Design review of the part built by this model. Coordinates are the model's own, in mm. Face numbers are marked on the shaded views. A direction names the side the tool comes from. Give positions to 0.01 mm unless a question says otherwise; leave off trailing zeros. Loops run counter-clockwise (first coordinate to the right, second up) from the corner with the lowest first, then second, coordinate; pieces in that order, holes last. Notation, with made-up numbers: (23, -23.5) -> (38, -23.5) arc R31 cw to (38, 4.5) -> close; hole circle Ø2 at (-25, 78.5). An arc over 180 degrees is marked (long way). Answer in a Markdown table with one row per item. Add a question column.
(1) Consider section C-C on x = -11.5. Write out the cut boundary in (y, z), then the cut area to 3 significant figures.
(2) For the marked faces 4, 5 and 6, list the 3-axis set-ups (+Z, -Z, +X, -X, +Y, -Y) from which the entire face can be reached by the end or side of a thin tool; tool diameter is ignored.
(3) Consider section A-A on z = 90. Write out the cut boundary in (x, y).
(4) Draft analysis for pull direction Y (two halves, no side actions). For the marked faces 1, 2 and 3, state which applies: +Y half, -Y half, draft (parallel to the pull), parting line (faces both ways), or undercut.
(5) Consider section D-D on z = 106. Write out the cut boundary in (x, y), then the cut area to 3 significant figures.
(6) For line 1 (Y direction, x = 34.5, z = 90.5); line 2 (Z direction, x = 6.5, y = -20); line 3 (X direction, y = 33, z = 91), list the stretches that pass through material, from the lowest coordinate up.
(7) Consider section B-B on y = 26.5. Write out the cut boundary in (x, z), then the cut area to 3 significant figures.
(8) For pin 1 (3 mm diameter, centred on x = -22.5, z = 48.5, fed in from -Y); pin 2 (11 mm diameter, centred on y = 30.5, z = 74.5, fed in from -X); pin 3 (3 mm diameter, centred on y = -30.5, z = 70.5, fed in from +X), all flat-tipped, find the tip position at first contact; note any pin that passes through.
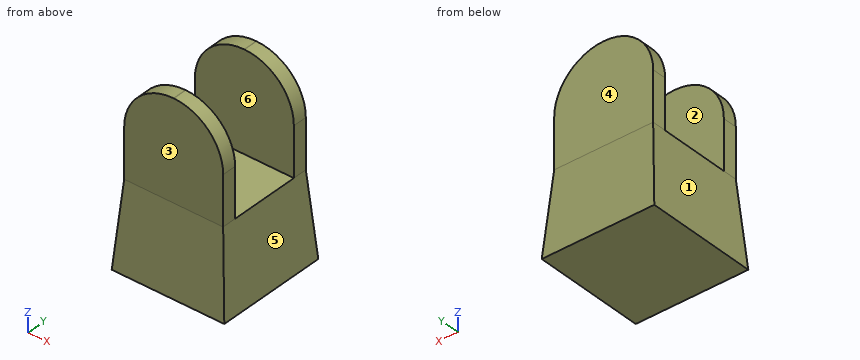
from build123d import *

# Parameters (mm, degrees)
SZKIC1_W                    = 80
SZKIC1_H                    = 80
DODANIE_WYCI_GNI_CIE1_DEPTH = 60
DODANIE_WYCI_GNI_CIE1_TAPER = 4.6
SZKIC6_W                    = 70.345029246
SZKIC6_H                    = 70.345029246
DODANIE_WYCI_GNI_CIE2_DEPTH = 70
ZAOKR_GLENIE3_R             = 35
ZAOKR_GLENIE4_R             = 35
SZKIC7_W                    = 70.345029246
SZKIC7_H                    = 50
WYTNIJ_WYCI_GNI_CIE3_DEPTH  = 70


with BuildPart() as part:
    # Szkic1 → Dodanie-wyciągnięcie1 (new body)
    with BuildSketch(Plane.XY):
        Rectangle(SZKIC1_W, SZKIC1_H)
    extrude(amount=DODANIE_WYCI_GNI_CIE1_DEPTH, taper=DODANIE_WYCI_GNI_CIE1_TAPER)

    # Szkic6 → Dodanie-wyciągnięcie2 (add)
    with BuildSketch(Plane.XY.offset(60)):
        Rectangle(SZKIC6_W, SZKIC6_H)
    extrude(amount=DODANIE_WYCI_GNI_CIE2_DEPTH)

    # Zaokrąglenie3
    zaokr_glenie3_edges = [part.edges().sort_by_distance(p)[0] for p in [
        (-35.172514623, 0, 130),
    ]]
    fillet(zaokr_glenie3_edges, radius=ZAOKR_GLENIE3_R)

    # Zaokrąglenie4
    zaokr_glenie4_edges = [part.edges().sort_by_distance(p)[0] for p in [
        (35.172514623, 0, 130),
    ]]
    fillet(zaokr_glenie4_edges, radius=ZAOKR_GLENIE4_R)

    # Szkic7 → Wytnij-wyciągnięcie3 (cut)
    with BuildSketch(Plane.XY.offset(130)):
        Rectangle(SZKIC7_W, SZKIC7_H)
    extrude(amount=-WYTNIJ_WYCI_GNI_CIE3_DEPTH, mode=Mode.SUBTRACT)


solid = part.part
Values follow:
| question | item | result |
|---|---|---|
| 1 | outline | (-40, 0) -> (40, 0) -> (35.17, 60) -> (35.17, 128.12) -> (25, 128.12) -> (25, 60) -> (-25, 60) -> (-25, 128.12) -> (-35.17, 128.12) -> (-35.17, 60) -> close |
| 1 | area | 5,900 mm2 |
| 2 | face 4 | +Z, +X, -X, +Y |
| 2 | face 5 | +Z, +X, +Y, -Y |
| 2 | face 6 | +Z, +X, -X |
| 3 | outline | (-35.17, -35.17) -> (35.17, -35.17) -> (35.17, -25) -> (-35.17, -25) -> close; (-35.17, 25) -> (35.17, 25) -> (35.17, 35.17) -> (-35.17, 35.17) -> close |
| 4 | face 1 | draft |
| 4 | face 2 | undercut |
| 4 | face 3 | -Y half |
| 5 | outline | (-33.4, -35.17) -> (33.4, -35.17) -> (33.4, -25) -> (-33.4, -25) -> close; (-33.4, 25) -> (33.4, 25) -> (33.4, 35.17) -> (-33.4, 35.17) -> close |
| 5 | area | 1,360 mm2 |
| 6 | line 1 | -35.17 to -25, 25 to 35.17 |
| 6 | line 2 | 0 to 60 |
| 6 | line 3 | -35.17 to 35.17 |
| 7 | outline | (-40, 0) -> (40, 0) -> (35.17, 60) -> (35.17, 95) arc R35 ccw to (0.17, 130) -> (-0.17, 130) arc R35 ccw to (-35.17, 95) -> (-35.17, 60) -> close |
| 7 | area | 8,910 mm2 |
| 8 | pin 1 | y = -36.22 |
| 8 | pin 2 | x = -35.17 |
| 8 | pin 3 | x = 35.17 |
